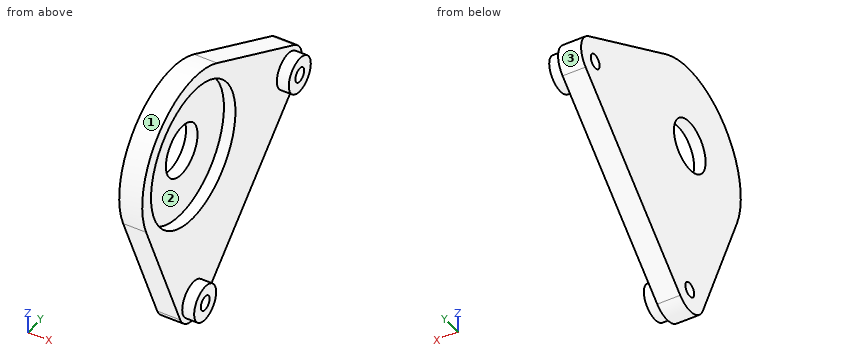
```python
from build123d import *

# Parameters (mm, degrees)
SKETCH1_R           = 14.5
SKETCH1_R_2         = 12
SKETCH1_R_3         = 4
SKETCH1_R_4         = 1.25
SKETCH1_R_5         = 3.125
BOSS_EXTRUDE1_DEPTH = 4
SKETCH1_3_R         = 3.125
SKETCH1_3_R_2       = 1.25
BOSS_EXTRUDE2_DEPTH = 6.08
SKETCH1_4_R         = 12
SKETCH1_4_R_2       = 4.5
BOSS_EXTRUDE3_DEPTH = 2


with BuildPart() as part:
    # Sketch1 → Boss-Extrude1 (new body)
    # profile 1 of 6: a face of its own
    with BuildSketch(Plane(origin=(0, 0, 0), x_dir=(0, 0, -1), z_dir=(1, 0, 0))):
        Circle(SKETCH1_R)
        Circle(SKETCH1_R_2, mode=Mode.SUBTRACT)
    # profile 2 of 6: a face of its own
    with BuildSketch(Plane(origin=(0, 0, 0), x_dir=(0, 0, -1), z_dir=(1, 0, 0))):
        with BuildLine():
            ThreePointArc((6.353205054, 26.897256848), (1.389400085, 23.015107961), (-1.182334937, 28.768074042))
            Line((-1.182334937, 28.768074042), (-12.816332467, 6.781712327))
            ThreePointArc((-12.816332467, 6.781712327), (3.493793012, 14.072789716), (14.5, 0))
            ThreePointArc((14.5, 0), (12.061665521, -8.04774657), (5.566727605, -13.388858942))
            Line((5.566727605, -13.388858942), (28.885648995, -3.693478329))
            ThreePointArc((28.885648995, -3.693478329), (23.441232053, 0.849431066), (30.280045487, 2.723019178))
            Line((30.280045487, 2.723019178), (5.283250541, 29.620276026))
            ThreePointArc((5.283250541, 29.620276026), (6.076119366, 28.360099638), (6.353205054, 26.897256848))
        make_face()
    # profile 3 of 6: a face of its own
    with BuildSketch(Plane(origin=(0, 0, 0), x_dir=(0, 0, -1), z_dir=(1, 0, 0))):
        with Locations((2.353205054, 26.897256848)):
            Circle(SKETCH1_R_3)
        with Locations((2.353205054, 26.897256848)):
            Circle(SKETCH1_R_4, mode=Mode.SUBTRACT)
    # profile 4 of 6: a face of its own
    with BuildSketch(Plane(origin=(0, 0, 0), x_dir=(0, 0, -1), z_dir=(1, 0, 0))):
        with Locations((27.35, 0)):
            Circle(SKETCH1_R_3)
        with Locations((27.35, 0)):
            Circle(SKETCH1_R_4, mode=Mode.SUBTRACT)
    # profile 5 of 6: a face of its own
    with BuildSketch(Plane(origin=(0, 0, 0), x_dir=(0, 0, -1), z_dir=(1, 0, 0))):
        with Locations((2.353205054, 26.897256848)):
            Circle(SKETCH1_R_5)
        with Locations((2.353205054, 26.897256848)):
            Circle(SKETCH1_R_4, mode=Mode.SUBTRACT)
    # profile 6 of 6: a face of its own
    with BuildSketch(Plane(origin=(0, 0, 0), x_dir=(0, 0, -1), z_dir=(1, 0, 0))):
        with Locations((27.35, 0)):
            Circle(SKETCH1_R_5)
        with Locations((27.35, 0)):
            Circle(SKETCH1_R_4, mode=Mode.SUBTRACT)
    extrude(amount=BOSS_EXTRUDE1_DEPTH)

    # Sketch1_3 → Boss-Extrude2 (add)
    # profile 1 of 2: a face of its own
    with BuildSketch(Plane(origin=(0, 0, 0), x_dir=(0, 0, -1), z_dir=(1, 0, 0))):
        with Locations((2.353205054, 26.897256848)):
            Circle(SKETCH1_3_R)
        with Locations((2.353205054, 26.897256848)):
            Circle(SKETCH1_3_R_2, mode=Mode.SUBTRACT)
    # profile 2 of 2: a face of its own
    with BuildSketch(Plane(origin=(0, 0, 0), x_dir=(0, 0, -1), z_dir=(1, 0, 0))):
        with Locations((27.35, 0)):
            Circle(SKETCH1_3_R)
        with Locations((27.35, 0)):
            Circle(SKETCH1_3_R_2, mode=Mode.SUBTRACT)
    extrude(amount=BOSS_EXTRUDE2_DEPTH)

    # Sketch1_4 → Boss-Extrude3 (add)
    with BuildSketch(Plane(origin=(0, 0, 0), x_dir=(0, 0, -1), z_dir=(1, 0, 0))):
        Circle(SKETCH1_4_R)
        Circle(SKETCH1_4_R_2, mode=Mode.SUBTRACT)
    extrude(amount=BOSS_EXTRUDE3_DEPTH)


solid = part.part
```
Could you check a few things on this model? Use its own coordinates, in mm. Face numbers are marked on the shaded views. Coordinates: 2 decimals unless noted, no trailing zeros. Loops run counter-clockwise (first coordinate to the right, second up) from the corner with the lowest first, then second, coordinate; pieces in that order, holes last.
1) Thinking about a two-plate mould opening in Y: for the marked faces 1, 2 and 3, which applies, released by +Y, released by -Y, zero draft, split by the parting line, or undercut?
Reported:
face 1: split by the parting line
face 2: undercut
face 3: released by +Y
2) Imagine slicing it at C-C (z = -27.35). List the corners of the cut face in (x, y) for me (3 decimals), and give its area (3 significant figures).
Reported:
outline: (0, -4.332) - (4, -4.332) - (4, -3.125) - (6.08, -3.125) - (6.08, -1.25) - (0, -1.25) - close; (0, 1.25) - (6.08, 1.25) - (6.08, 3.125) - (4, 3.125) - (4, 5.876) - (0, 5.876) - close
area: 38.6 mm2
3) Imagine slicing it at A-A (y = 0). List the corners of the cut face in (x, z) for me (3 decimals).
Reported:
outline: (0, -31.35) - (4, -31.35) - (4, -30.475) - (6.08, -30.475) - (6.08, -28.6) - (0, -28.6) - close; (0, -26.1) - (6.08, -26.1) - (6.08, -24.225) - (4, -24.225) - (4, -12) - (2, -12) - (2, -4.5) - (0, -4.5) - close; (0, 4.5) - (2, 4.5) - (2, 12) - (4, 12) - (4, 14.5) - (0, 14.5) - close
4) Imagine slicing it at D-D (z = 10). List the corners of the cut face in (x, y) for me.
Reported:
outline: (0, -10.5) - (4, -10.5) - (4, -6.63) - (2, -6.63) - (2, 6.63) - (4, 6.63) - (4, 12.1) - (0, 12.1) - close
5) Will these pins go through, and if not, where does the flat tip stop? pin 1 Ø19 at (y, z) = (4.5, 4.5) entering from +X; pin 2 Ø1.5 at (x, z) = (0.5, 1.5) entering from -Y; pin 3 Ø1.5 at (x, z) = (2.5, -6) entering from -Y.
Reported:
pin 1: stops at x = 4
pin 2: stops at y = -14.48
pin 3: stops at y = -13.52
6) Please list where these lines run through material, in increasing order: line 1 along X through (y, z) = (7, -22.5); line 2 along Z through (x, y) = (2.5, -4); line 3 along Y through (x, z) = (1.25, 0.5).
Reported:
line 1: x = 0 to 4
line 2: z = -28.15 to -11.31, 11.31 to 13.94
line 3: y = -14.49 to -4.47, 4.47 to 29.7
7) Imagine slicing it at B-B (x = 1.25). List the corners of the cut face in (y, z) for me.
Reported:
outline: (-13.39, -5.57) - (-3.69, -28.89) arc R4 ccw to (2.72, -30.28) - (29.62, -5.28) arc R4 ccw to (28.77, 1.18) - (6.78, 12.82) arc R14.5 ccw to start; hole circle Ø9 at (0, 0); hole circle Ø2.5 at (0, -27.35); hole circle Ø2.5 at (26.9, -2.35)
